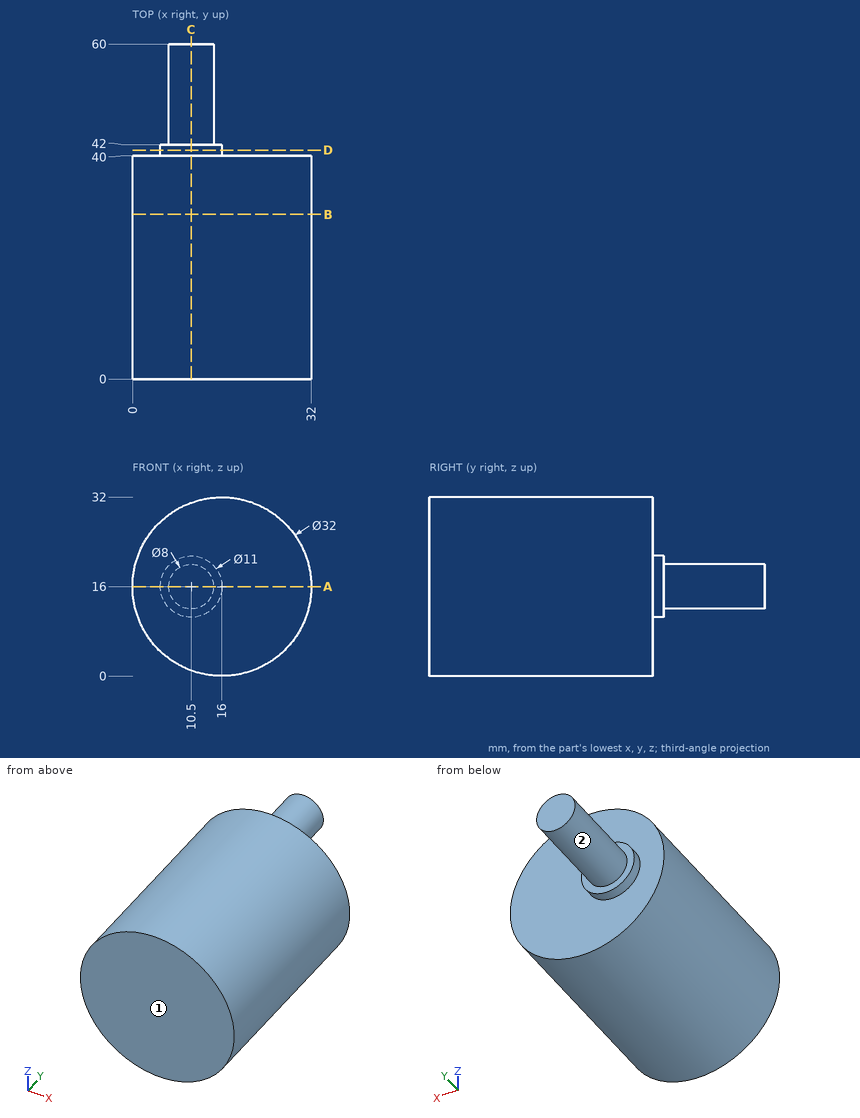
Geometry check sheet. Reference: drawing and pictorial views, mm from the part's lowest x, y, z. A direction names the side the tool comes from. Round coordinates to 2 decimals unless told otherwise and drop trailing zeros. Loops run counter-clockwise (first coordinate to the right, second up) from the corner with the lowest first, then second, coordinate; pieces in that order, holes last. Notation, with made-up numbers: (-22.5, 21) - (3.5, 21) arc R8 cw to (3.5, 30) - close; hole circle Ø9 at (81, -7.5). An arc over 180 degrees is marked (long way). Use a Markdown table: item, result.
Q1. Material ranges on line 1 (Y direction, x = 10, z = 24.5); line 2 (Z direction, x = 26, y = 17); line 3 (Y direction, x = 12, z = 11), recorded low to high.
Solutions:
| item | result |
|---|---|
| line 1 | y = 0 to 40 |
| line 2 | z = 3.51 to 28.49 |
| line 3 | y = 0 to 42 |
Q2. Go/stop test with flat-tipped pins: P1, Ø8, axis at x = 7, y = 31.5, coming from the -Z side; P2, Ø12, axis at y = 51, z = 8.5, coming from the +X side; P3, Ø1, axis at y = 46.5, z = 17, coming from the +X side. Record where each tip stops, or that it passes through.
Solutions:
| item | result |
|---|---|
| P1 | stops at z = 0.8 |
| P2 | stops at x = 14.21 |
| P3 | stops at x = 14.47 |
Q3. Cross-section at B-B on y = 29.5. Record the cut outline in (x, z).
Solutions:
| item | result |
|---|---|
| outline | circle Ø32 at (16, 16) |
Q4. Cross-section at C-C on x = 10.5. Record the cut outline in (y, z).
Solutions:
| item | result |
|---|---|
| outline | (0, 0.98) - (40, 0.98) - (40, 10.5) - (42, 10.5) - (42, 12) - (60, 12) - (60, 20) - (42, 20) - (42, 21.5) - (40, 21.5) - (40, 31.02) - (0, 31.02) - close |
Q5. Cross-section at A-A on z = 16. Record the cut outline in (x, y), plus the area to 3 significant figures.
Solutions:
| item | result |
|---|---|
| outline | (0, 0) - (32, 0) - (32, 40) - (16, 40) - (16, 42) - (14.5, 42) - (14.5, 60) - (6.5, 60) - (6.5, 42) - (5, 42) - (5, 40) - (0, 40) - close |
| area | 1,450 mm2 |
Q6. Cross-section at D-D on y = 41. Record the cut outline in (x, z), plus the area to 3 significant figures.
Solutions:
| item | result |
|---|---|
| outline | circle Ø11 at (10.5, 16) |
| area | 95.0 mm2 |
Q7. Access from +Z, -Z, +X, -X, +Y, -Y to the whole of each face (thin tool, end or side, straight path). Record for the marked faces 1 and 2.
Solutions:
| item | result |
|---|---|
| face 1 | +Z, -Z, +X, -X, -Y |
| face 2 | +Y |
